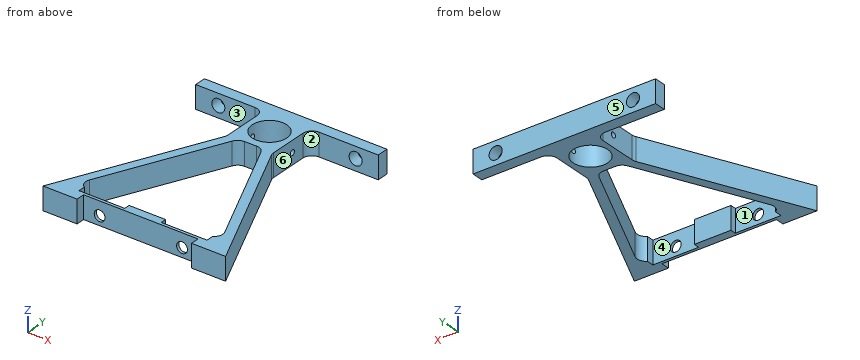
```python
from build123d import *

# Parameters (mm, degrees)
SKETCH3_R               = 9.5885
BOSS_EXTRUDE1_DEPTH     = 12.7
SKETCH4_R               = 3.614257139
CUT_EXTRUDE1_DEPTH      = 6.35
CUT_EXTRUDE2_START      = -12.7
CUT_EXTRUDE2_OUTLINE_R  = 1.5
CUT_EXTRUDE2_DEPTH      = 25.4
CUT_EXTRUDE3_DEPTH      = 126.664030474
CUT_EXTRUDE3_DEPTH_BACK = 126.664030474
SKETCH8_W               = 25.4
SKETCH8_H               = 5.08
SKETCH9_R               = 3
CUT_EXTRUDE4_DEPTH      = 123.783240632


# Read off the part's stored shape, not the designer's step: Cut-Extrude2
with BuildPart() as part:
    # Sketch3 → Boss-Extrude1 (new body)
    with BuildSketch(Plane.XY):
        with BuildLine():
            Line((50.652428891, 3.175), (-50.652428891, 3.175))
            Line((-50.652428891, 3.175), (-50.652428891, -3.175))
            Line((-50.652428891, -3.175), (-17.78, -3.175))
            ThreePointArc((-17.78, -3.175), (-14.187897552, -4.662897552), (-12.7, -8.255))
            Line((-12.7, -8.255), (-12.7, -29.595434395))
            ThreePointArc((-12.7, -29.595434395), (-12.814872576, -30.66963627), (-13.154295145, -31.69525691))
            Line((-13.154295145, -31.69525691), (-50.652428891, -114.3))
            Line((-50.652428891, -114.3), (-31.75, -114.3))
            Line((-31.75, -114.3), (-31.75, -109.5375))
            Line((-31.75, -109.5375), (31.75, -109.5375))
            Line((31.75, -109.5375), (31.75, -114.3))
            Line((31.75, -114.3), (50.652428891, -114.3))
            Line((50.652428891, -114.3), (13.154295145, -31.69525691))
            ThreePointArc((13.154295145, -31.69525691), (12.814872576, -30.66963627), (12.7, -29.595434395))
            Line((12.7, -29.595434395), (12.7, -8.255))
            ThreePointArc((12.7, -8.255), (14.187897552, -4.662897552), (17.78, -3.175))
            Line((17.78, -3.175), (50.652428891, -3.175))
            Line((50.652428891, -3.175), (50.652428891, 3.175))
        make_face()
        with Locations((0, -15.875)):
            Circle(SKETCH3_R, mode=Mode.SUBTRACT)
        with BuildLine():
            Line((-7.97501727, -32.575611881), (-37.490421301, -97.595177486))
            ThreePointArc((-37.490421301, -97.595177486), (-37.135167146, -102.446299841), (-32.864716446, -104.775))
            Line((-32.864716446, -104.775), (0, -104.775))
            Line((0, -104.775), (32.864716446, -104.775))
            ThreePointArc((32.864716446, -104.775), (37.135167146, -102.446299841), (37.490421301, -97.595177486))
            Line((37.490421301, -97.595177486), (7.97501727, -32.575611881))
            ThreePointArc((7.97501727, -32.575611881), (6.100612256, -30.404983695), (3.349312415, -29.595434395))
            Line((3.349312415, -29.595434395), (-3.349312415, -29.595434395))
            ThreePointArc((-3.349312415, -29.595434395), (-6.100612256, -30.404983695), (-7.97501727, -32.575611881))
        make_face(mode=Mode.SUBTRACT)
    extrude(amount=BOSS_EXTRUDE1_DEPTH)

    # Sketch4 → Cut-Extrude1 (cut)
    with BuildSketch(Plane(origin=(0, 3.175, 0), x_dir=(1, 0, 0), z_dir=(0, 1, 0))):
        with Locations(Location((-38.1, -6.35, 0), (0, 0, 180))):
            Circle(SKETCH4_R)
        with Locations(Location((38.1, -6.35, 0), (0, 0, 180))):
            Circle(SKETCH4_R)
    extrude(amount=-CUT_EXTRUDE1_DEPTH, mode=Mode.SUBTRACT)

    # Cut-Extrude2 outline → Cut-Extrude2 (cut)
    with BuildSketch(Plane.YZ.offset(CUT_EXTRUDE2_START)):
        with Locations((-15.883331584, 6.35)):
            Circle(CUT_EXTRUDE2_OUTLINE_R)
    extrude(amount=CUT_EXTRUDE2_DEPTH, mode=Mode.SUBTRACT)

    # Sketch8 → Cut-Extrude3 (cut, two sides: drawn at the far end of the back side and taken through both)
    with BuildSketch(Plane.XY.offset(12.7).offset(-CUT_EXTRUDE3_DEPTH_BACK)):
        with Locations((-22.86, -105.41)):
            Rectangle(SKETCH8_W, SKETCH8_H)
        with Locations((22.86, -105.41)):
            Rectangle(SKETCH8_W, SKETCH8_H)
    extrude(amount=CUT_EXTRUDE3_DEPTH + CUT_EXTRUDE3_DEPTH_BACK, mode=Mode.SUBTRACT)

    # Sketch9 → Cut-Extrude4 (cut, through all)
    with BuildSketch(Plane(origin=(0, -107.95, 0), x_dir=(1, 0, 0), z_dir=(0, 1, 0))):
        with Locations(Location((-22.86, -5.08, 0), (0, 0, 270))):
            Circle(SKETCH9_R)
        with Locations((22.86, -5.08)):
            Circle(SKETCH9_R)
    extrude(amount=-CUT_EXTRUDE4_DEPTH, mode=Mode.SUBTRACT)


solid = part.part
```
Model file for the job. Use its own axes, mm. Face numbers are marked on the shaded views. A direction names the side the tool comes from. Coordinates: 2 decimals unless noted, no trailing zeros. Write each loop counter-clockwise with the first axis right and the second up, starting at its lowest first coordinate (ties: lowest second). Pieces come first, ordered by that corner, then holes. Notation, with made-up numbers: (79.25, 19) - (104.25, 19) arc R32 cw to (104.25, 51) - close; hole circle Ø5 at (8, 28.5). An arc over 180 degrees is marked (long way). Use a Markdown table: item, result. Add a question column.
Item 1: 3-axis set-ups, long thin cutter, end or side, ignore diameter. For the marked faces 1, 2 and 3: which of +Z, -Z, +X, -X, +Y, -Y reach the whole face in a straight line?
Item 2: Band-saw the part on A-A, the plane x = -27.5. Give the number of separate pieces and of enclosed holes in the cut face, and give its area (3 significant figures).
Item 3: Two-plate mould, pull along X, no slides. Class the marked faces 4, 5 and 6: pulls with the +X half, pulls with the -X half, needs draft (parallel to the pull), parting line crosses it, or undercut.
Item 4: Drop flat-ended pins along their axis: pin 1 (2 mm diameter, centred on x = -8.5, z = 6.5, fed in from -Y); pin 2 (4.5 mm diameter, centred on y = -106.5, z = 5, fed in from +X); pin 3 (12 mm diameter, centred on x = 23, y = -91, fed in from -Z); pin 4 (5.5 mm diameter, centred on x = -22.86, z = 5.08, fed in from -Y). Give the stop position or say it passes through.
Item 5: Band-saw the part on B-B, the plane y = -81. Write the cut outline in (x, z), and give its area (3 significant figures).
Item 6: Drill centre lines: line 1 along Z through (x, y) = (38, 0); line 2 along Y through (x, z) = (-34, 1) (3 decimals); line 3 along X through (y, z) = (-108.4, 5.08). Where is each one in solid material? Low to high.
A:
| question | item | result |
|---|---|---|
| 1 | face 1 | +Z, -Z |
| 1 | face 2 | +Z, -Z, +X |
| 1 | face 3 | +Z, -Z, -X |
| 2 | separate pieces | 3 |
| 2 | enclosed holes | 0 |
| 2 | area | 257 mm² |
| 3 | face 4 | undercut |
| 3 | face 5 | needs draft |
| 3 | face 6 | pulls with the +X half |
| 4 | pin 1 | stops at y = -109.54 |
| 4 | pin 2 | stops at x = 48.13 |
| 4 | pin 3 | passes through |
| 4 | pin 4 | stops at y = -71.42 |
| 5 | outline | (-35.54, 0) - (-29.96, 0) - (-29.96, 12.7) - (-35.54, 12.7) - close; (29.96, 0) - (35.54, 0) - (35.54, 12.7) - (29.96, 12.7) - close |
| 5 | area | 142 mm² |
| 6 | line 1 | z = 0 to 2.74, 9.96 to 12.7 |
| 6 | line 2 | y = -114.3 to -107.95, -89.906 to -77.616, -3.175 to 3.175 |
| 6 | line 3 | x = -47.97 to -25.86, -19.86 to 19.86, 25.86 to 47.97 |
